Geometry check sheet. Reference: the model listing, model coordinates, mm. Coordinates: 2 decimals unless noted, no trailing zeros. Loops run counter-clockwise (first coordinate to the right, second up) from the corner with the lowest first, then second, coordinate; pieces in that order, holes last.
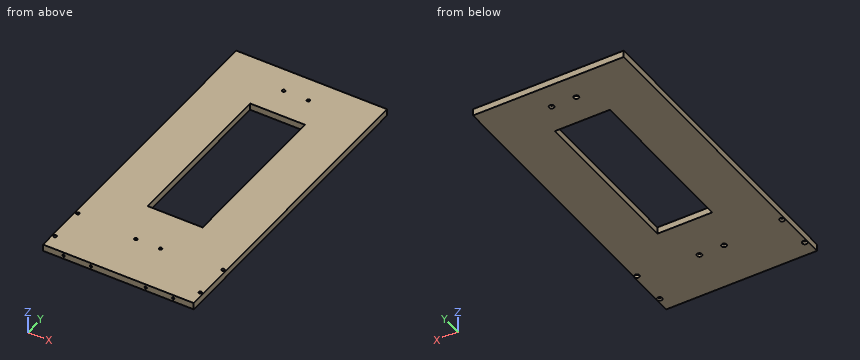
from build123d import *

# Parameters (mm, degrees)
SKETCH1_W               = 330
SKETCH1_H               = 680
BOSS_EXTRUDE1_DEPTH     = 15
CUT_EXTRUDE1_DEPTH      = 700.892848942
CUT_EXTRUDE1_DEPTH_BACK = 700.892848942
SKETCH2_R               = 3.3
SKETCH3_R               = 5.5
CUT_EXTRUDE3_DEPTH      = 6.5
CUT_EXTRUDE4_DEPTH      = 700.892848942
CUT_EXTRUDE4_DEPTH_BACK = 700.892848942
SKETCH4_R               = 3.3
SKETCH5_R               = 5.5
CUT_EXTRUDE6_DEPTH      = 6.5
SKETCH6_R               = 2.5
CUT_EXTRUDE8_DEPTH      = 15
CUT_EXTRUDE9_DEPTH      = 700.892848942
CUT_EXTRUDE9_DEPTH_BACK = 700.892848942
SKETCH7_W               = 120
SKETCH7_H               = 360


with BuildPart() as part:
    # Sketch1 → Boss-Extrude1 (new body)
    with BuildSketch(Plane.XY):
        with Locations((0, 340)):
            Rectangle(SKETCH1_W, SKETCH1_H)
    extrude(amount=BOSS_EXTRUDE1_DEPTH)

    # Sketch2 → Cut-Extrude1 (cut, two sides: drawn at the far end of the back side and taken through both)
    with BuildSketch(Plane.XY.offset(-CUT_EXTRUDE1_DEPTH_BACK)):
        with Locations((-27, 105)):
            Circle(SKETCH2_R)
        with Locations((-27, 625)):
            Circle(SKETCH2_R)
        with Locations((27, 105)):
            Circle(SKETCH2_R)
        with Locations((27, 625)):
            Circle(SKETCH2_R)
    extrude(amount=CUT_EXTRUDE1_DEPTH + CUT_EXTRUDE1_DEPTH_BACK, mode=Mode.SUBTRACT)

    # Sketch3 → Cut-Extrude3 (cut)
    with BuildSketch(Plane.XY):
        with Locations((-27, 105)):
            Circle(SKETCH3_R)
        with Locations((-27, 625)):
            Circle(SKETCH3_R)
        with Locations((27, 105)):
            Circle(SKETCH3_R)
        with Locations((27, 625)):
            Circle(SKETCH3_R)
    extrude(amount=CUT_EXTRUDE3_DEPTH, mode=Mode.SUBTRACT)

    # Sketch4 → Cut-Extrude4 (cut, two sides: drawn at the far end of the back side and taken through both)
    with BuildSketch(Plane.XY.offset(-CUT_EXTRUDE4_DEPTH_BACK)):
        with Locations((-159, 33)):
            Circle(SKETCH4_R)
        with Locations((-159, 113)):
            Circle(SKETCH4_R)
        with Locations((159, 33)):
            Circle(SKETCH4_R)
        with Locations((159, 113)):
            Circle(SKETCH4_R)
    extrude(amount=CUT_EXTRUDE4_DEPTH + CUT_EXTRUDE4_DEPTH_BACK, mode=Mode.SUBTRACT)

    # Sketch5 → Cut-Extrude6 (cut)
    with BuildSketch(Plane.XY):
        with Locations((-159, 33)):
            Circle(SKETCH5_R)
        with Locations((-159, 113)):
            Circle(SKETCH5_R)
        with Locations((159, 33)):
            Circle(SKETCH5_R)
        with Locations((159, 113)):
            Circle(SKETCH5_R)
    extrude(amount=CUT_EXTRUDE6_DEPTH, mode=Mode.SUBTRACT)

    # Sketch6 → Cut-Extrude8 (cut)
    with BuildSketch(Plane(origin=(0, 0, 0), x_dir=(1, 0, 0), z_dir=(0, 1, 0))):
        with Locations(Location((-120, -7.5, 0), (0, 0, 270))):
            Circle(SKETCH6_R)
        with Locations(Location((-60, -7.5, 0), (0, 0, 270))):
            Circle(SKETCH6_R)
        with Locations(Location((60, -7.5, 0), (0, 0, 270))):
            Circle(SKETCH6_R)
        with Locations(Location((120, -7.5, 0), (0, 0, 270))):
            Circle(SKETCH6_R)
    extrude(amount=CUT_EXTRUDE8_DEPTH, mode=Mode.SUBTRACT)

    # Sketch7 → Cut-Extrude9 (cut, two sides: drawn at the far end of the back side and taken through both)
    with BuildSketch(Plane.XY.offset(-CUT_EXTRUDE9_DEPTH_BACK)):
        with Locations((0, 380)):
            Rectangle(SKETCH7_W, SKETCH7_H)
    extrude(amount=CUT_EXTRUDE9_DEPTH + CUT_EXTRUDE9_DEPTH_BACK, mode=Mode.SUBTRACT)


solid = part.part
1) Section check B-B on x = -8. Record the cut outline in (y, z).
Data:
outline: (0, 0) - (200, 0) - (200, 15) - (0, 15) - close; (560, 0) - (680, 0) - (680, 15) - (560, 15) - close
2) Section check A-A on z = 12.5. Count the separate pieces of the cut face and the enclosed holes in it, and give its area (3 significant figures).
Data:
separate pieces: 1
enclosed holes: 9
area: 181,000 mm2
3) Material ranges on probe 1 along Y at (x, z) = (27, 2.5); probe 2 along X at (y, z) = (113, 10.75); probe 3 along X at (y, z) = (255, 10.75), recorded low to high.
Data:
probe 1: y = 0 to 99.5, 110.5 to 200, 560 to 619.5, 630.5 to 680
probe 2: x = -165 to -162.3, -155.7 to 155.7, 162.3 to 165
probe 3: x = -165 to -60, 60 to 165
4) Depth check by flat-ended pin: pin 1 (3 mm diameter, centred on x = -120, z = 7.5, fed in from -Y); pin 2 (10.5 mm diameter, centred on x = 159, y = 113, fed in from -Z). Enter the tip coordinate at first touch or a pass-through.
Data:
pin 1: stops at y = 15
pin 2: stops at z = 6.5
